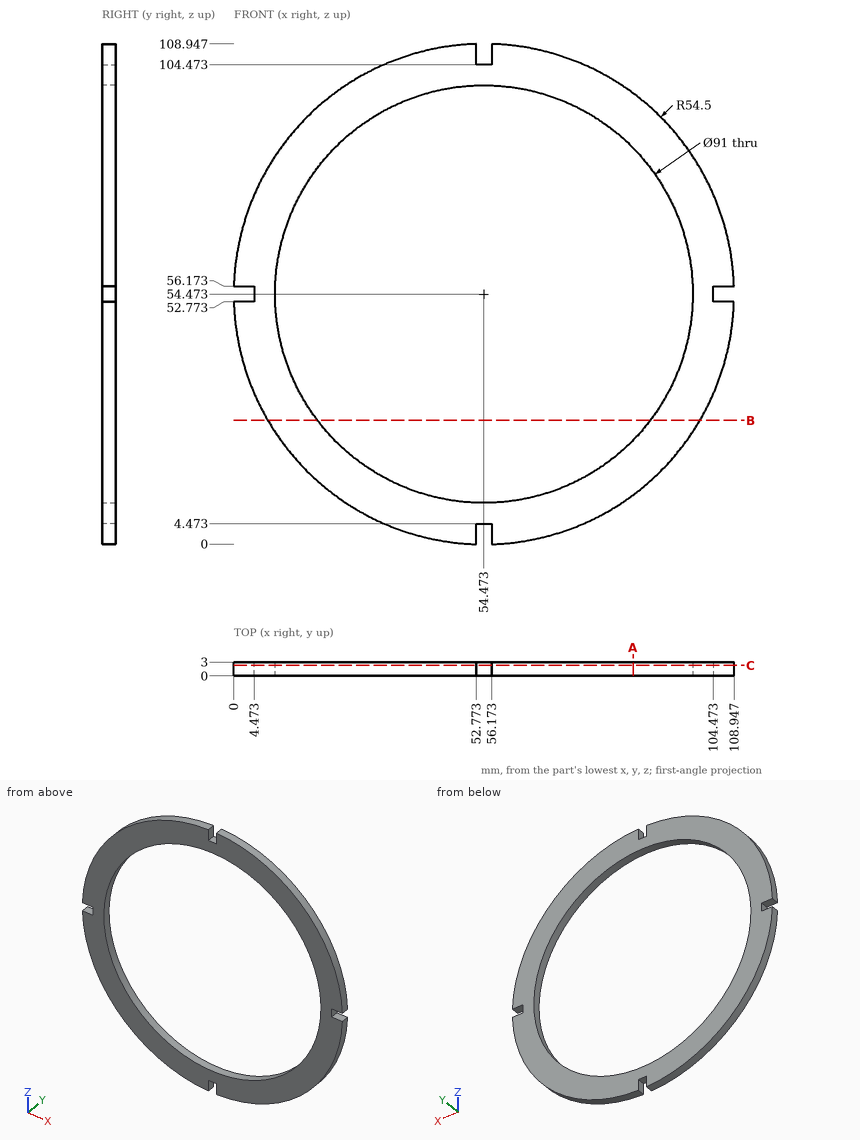
The drawing under review shows one solid part. Ordinate dimensions are in mm from its lowest x, y, z. Give positions to 0.01 mm unless a question says otherwise; leave off trailing zeros. Loops run counter-clockwise (first coordinate to the right, second up) from the corner with the lowest first, then second, coordinate; pieces in that order, holes last. Notation, with made-up numbers: M -32,6.25 L -13,6.25 A11 cw -13,18.25 Z; hole C 75,-10.75 d3. An arc over 180 degrees is marked long. Return JSON: item names as keys, results as strings. Group by question number.
Item 1: For probe 1 along X at (y, z) = (0.8, 71) (1 decimal); probe 2 along Z at (x, y) = (17, 2.25) (1 decimal); probe 3 along Z at (x, y) = (85, 2.5) (1 decimal), list the stretches that pass through material, from the lowest coordinate up.
Item 2: We need section C-C (y = 2.3). Give the boundary of the cut face in (x, z).
Item 3: We need section B-B (z = 27). Give the boundary of the cut face in (x, y) (1 decimal).
Item 4: Insertion check: pin 1 Ø1.5 at (y, z) = (1, 54) entering from +X; pin 2 Ø1.5 at (x, y) = (55, 2) entering from -Z; pin 3 Ø1.5 at (y, z) = (1, 54) entering from -X. Each pin has a flat end and moves straight along its axis. Give the tip position at first contact, or say it passes through.
Item 5: We need section A-A (x = 87). Give the boundary of the cut face in (y, z).
Output:
{
 "1": {"probe 1": "x = 2.5 to 12.1, 96.9 to 106.4", "probe 2": "z = 14.9 to 28.7, 80.3 to 94", "probe 3": "z = 9.3 to 20.7, 88.2 to 99.6"},
 "2": {"outline": "M 0,52.77 A54.5 ccw 52.77,0 L 52.77,4.47 L 56.17,4.47 L 56.17,0 A54.5 ccw 108.95,52.77 L 104.47,52.77 L 104.47,56.17 L 108.95,56.17 A54.5 ccw 56.17,108.95 L 56.17,104.47 L 52.77,104.47 L 52.77,108.95 A54.5 ccw 0,56.17 L 4.47,56.17 L 4.47,52.77 Z; hole C 54.47,54.47 d91"},
 "3": {"outline": "M 7.4,0 L 18.2,0 L 18.2,3 L 7.4,3 Z; M 90.7,0 L 101.5,0 L 101.5,3 L 90.7,3 Z"},
 "4": {"pin 1": "stops at x = 104.47", "pin 2": "stops at z = 4.47", "pin 3": "stops at x = 4.47"},
 "5": {"outline": "M 0,10.74 L 3,10.74 L 3,22.66 L 0,22.66 Z; M 0,86.29 L 3,86.29 L 3,98.2 L 0,98.2 Z"}
}
